```python
from build123d import *

# Parameters (mm, degrees)
F0_R      = 21
F1_DEPTH  = 39.2
F3_R      = 4
F4_DEPTH  = 22
F5_R      = 12.5
F6_DEPTH  = 2
F7_R      = 22.5
F8_DEPTH  = 66
F9_R      = 7.5
F10_DEPTH = 5
F11_R     = 2
F12_DEPTH = 5


with BuildPart() as f1:
    # F0 (on Front) → F1 (new body)
    with BuildSketch(Plane.XZ):
        Circle(F0_R)
    extrude(amount=F1_DEPTH)

    # F3 (on face) → F4 (join)
    with BuildSketch(Plane(origin=(0, 0, 0), x_dir=(-1, 0, 0), z_dir=(0, 1, 0))):
        Circle(F3_R)
    extrude(amount=F4_DEPTH)

    # F5 (on face) → F6 (join)
    with BuildSketch(Plane(origin=(0, 0, 0), x_dir=(-1, 0, 0), z_dir=(0, 1, 0))):
        Circle(F5_R)
    extrude(amount=F6_DEPTH)

    # F7 (on face) → F8 (join)
    with BuildSketch(Plane.XZ.offset(39.2)):
        Circle(F7_R)
    extrude(amount=F8_DEPTH)

    # F9 (on face) → F10 (join)
    with BuildSketch(Plane.XZ.offset(105.2)):
        Circle(F9_R)
    extrude(amount=F10_DEPTH)

    # F11 (on face) → F12 (cut)
    with BuildSketch(Plane(origin=(0, 0, 0), x_dir=(-1, 0, 0), z_dir=(0, 1, 0))):
        with Locations((-17.5, 0)):
            Circle(F11_R)
        with Locations((0, 17.5)):
            Circle(F11_R)
        with Locations((17.5, 0)):
            Circle(F11_R)
        with Locations((0, -17.5)):
            Circle(F11_R)
    extrude(amount=-F12_DEPTH, mode=Mode.SUBTRACT)


solid = f1.part
```
CAD build for the part. Positions are in the model's coordinates, mm. A direction names the side the tool comes from. Round coordinates to 2 decimals unless told otherwise and drop trailing zeros. Loops run counter-clockwise (first coordinate to the right, second up) from the corner with the lowest first, then second, coordinate; pieces in that order, holes last. Notation, with made-up numbers: M 77,-37 L 111,-37 A21 ccw 111,-15 Z; hole C -36,31.25 d8. An arc over 180 degrees is marked long. Return JSON: item names as keys, results as strings. Group by question number.
(1) Mould opens along Z. For faces 1 (the flat face through (0, -110.2, 0)), 2 (the cylindrical face through (-15.9, -2.5, -1.2)), 3 (the cylindrical face through (-11.923, 0.986, 3.755)) say: +Z half, -Z half, draft (parallel to the pull), parting line (faces both ways), or undercut.
(2) Wall check: probe 1 along Z at (x, y) = (0, -2); probe 2 along Y at (x, z) = (-9, 1); probe 3 along Y at (x, z) = (-2, -14.5). Give the ranges that are in metal, low to high. Write a range as [from, to].
(3) Saw through at D-D, the plane y = -26. List the corners of the cut face in (x, z).
(4) Drop flat-ended pins along their axis: P1, Ø2, axis at y = -64, z = 13.5, coming from the +X side; P2, Ø3, axis at x = 0.5, z = -18, coming from the +Y side; P3, Ø12, axis at x = 8.5, y = -52.5, coming from the -Z side. Give the stop position or say it passes through.
(5) Saw through at C-C, the plane y = 10.5. List the corners of the cut face in (x, z), and give its area (3 significant figures).
(6) Tool access for faces 4 (the cylindrical face through (-7.493, -107.665, 0.33)), 5 (the cylindrical face through (0.26, -2.465, -15.517)), 6 (the cylindrical face through (10.382, -71.738, -19.961)): list every direction of +Z, -Z, +X, -X, +Y, -Y with a clear straight run to the whole face (end or side of a thin tool).
(7) Saw through at B-B, the plane x = 0. List the corners of the cut face in (y, z), and give its area (3 significant figures).
(8) Saw through at A-A, the plane z = 0. List the corners of the cut face in (x, y).
Answer list:
{
 "1": {"face 1": "draft", "face 2": "undercut", "face 3": "parting line"},
 "2": {"probe 1": "[-21, -19.5], [-15.5, 15.5], [19.5, 21]", "probe 2": "[-105.2, 2]", "probe 3": "[-105.2, 0]"},
 "3": {"outline": "C 0,0 d42"},
 "4": {"P1": "x = 18.71", "P2": "y = 0", "P3": "z = -22.36"},
 "5": {"outline": "C 0,0 d8", "area": "50.3 mm2"},
 "6": {"face 4": "-Y", "face 5": "+Y", "face 6": "+Y, -Y"},
 "7": {"outline": "M -110.2,-7.5 L -105.2,-7.5 L -105.2,-22.5 L -39.2,-22.5 L -39.2,-21 L 0,-21 L 0,-19.5 L -5,-19.5 L -5,-15.5 L 0,-15.5 L 0,-12.5 L 2,-12.5 L 2,-4 L 22,-4 L 22,4 L 2,4 L 2,12.5 L 0,12.5 L 0,15.5 L -5,15.5 L -5,19.5 L 0,19.5 L 0,21 L -39.2,21 L -39.2,22.5 L -105.2,22.5 L -105.2,7.5 L -110.2,7.5 Z", "area": "4,860 mm2"},
 "8": {"outline": "M -22.5,-105.2 L -7.5,-105.2 L -7.5,-110.2 L 7.5,-110.2 L 7.5,-105.2 L 22.5,-105.2 L 22.5,-39.2 L 21,-39.2 L 21,0 L 19.5,0 L 19.5,-5 L 15.5,-5 L 15.5,0 L 12.5,0 L 12.5,2 L 4,2 L 4,22 L -4,22 L -4,2 L -12.5,2 L -12.5,0 L -15.5,0 L -15.5,-5 L -19.5,-5 L -19.5,0 L -21,0 L -21,-39.2 L -22.5,-39.2 Z"}
}
